```python
from build123d import *

# Parameters (mm, degrees)
SKETCH008_R       = 15
PAD004_DEPTH      = 3
PAD005_DEPTH      = 2
PAD005_DEPTH_BACK = 2
FILLET_R          = 2


with BuildPart() as part:
    # Sketch008 → Pad004 (new body)
    with BuildSketch(Plane.XY):
        Circle(SKETCH008_R)
    extrude(amount=PAD004_DEPTH)

    # Sketch009 → Pad005 (join, two sides)
    with BuildSketch(Plane.XZ) as pad005_sk:
        Polygon((-2, 0), (2, 0), (2, 24), (13.294118, 45.176471), (9.764706, 47.058824), (-2, 25), align=None)
    extrude(amount=PAD005_DEPTH)
    extrude(pad005_sk.sketch, amount=-PAD005_DEPTH_BACK)

    # Fillet
    fillet_edges = [part.edges().sort_by_distance(p)[0] for p in [
        (-15, 0, 3),
    ]]
    fillet(fillet_edges, radius=FILLET_R)


solid = part.part
```
For this review, take the finished solid that the model builds, in its own axes (mm). A direction names the side the tool comes from. Round coordinates to 2 decimals unless told otherwise and drop trailing zeros. Loops run counter-clockwise (first coordinate to the right, second up) from the corner with the lowest first, then second, coordinate; pieces in that order, holes last.
Q1. Insertion check: pin 1 Ø8 at (x, z) = (-2, 8.5) entering from +Y; pin 2 Ø4.5 at (x, z) = (3.5, 19) entering from -Y; pin 3 Ø1.2 at (y, z) = (-0.5, 17) entering from -X. Each pin has a flat end and moves straight along its axis. Give the tip position at first contact, or say it passes through.
Result sheet:
pin 1: stops at y = 2
pin 2: stops at y = -2
pin 3: stops at x = -2
Q2. Mouldability with a two-part tool opening along Z and no side actions: class faces 1 (the face through (3.965, 0.028, 36.184)), 2 (the face through (2, 2, 25)), 3 (the face through (2, 0, 13)) as +Z half, -Z half, draft (parallel to the pull), parting line (faces both ways), or undercut.
Result sheet:
face 1: +Z half
face 2: draft
face 3: undercut
Q3. Add section D-D on z = 30. Write out the cut boundary in (x, y).
Result sheet:
outline: (0.67, -2) - (5.2, -2) - (5.2, 2) - (0.67, 2) - close
Q4. Add section B-B on y = 0. Write out the cut boundary in (x, z).
Result sheet:
outline: (-15, 0) - (15, 0) - (15, 1) arc R2 ccw to (13, 3) - (2, 3) - (2, 24) - (13.29, 45.18) - (9.76, 47.06) - (-2, 25) - (-2, 3) - (-13, 3) arc R2 ccw to (-15, 1) - close
Q5. Add section C-C on z = 11.5. Write out the cut boundary in (x, y), plus the area to 3 significant figures.
Result sheet:
outline: (-2, -2) - (2, -2) - (2, 2) - (-2, 2) - close
area: 16.0 mm2
Q6. To check wall thickness, follow line 1 along Z through (x, y) = (-7.5, -5.5); line 2 along Y through (x, z) = (10, 43); line 3 along Z through (x, y) = (9, -0.25) (3 decimals). State the ranges of each line that lie inside material, in increasing order.
Result sheet:
line 1: z = 0 to 3
line 2: y = -2 to 2
line 3: z = 0 to 3, 37.125 to 45.625
Q7. Add section A-A on x = 0. Write out the cut boundary in (y, z).
Result sheet:
outline: (-15, 0) - (15, 0) - (15, 1) arc R2 ccw to (13, 3) - (2, 3) - (2, 28.75) - (-2, 28.75) - (-2, 3) - (-13, 3) arc R2 ccw to (-15, 1) - close
Q8. Machinability: for faces 4 (the face through (7.57, 0.03, 34.44)), 5 (the face through (11.554, 0.028, 46.104)), 6 (the face through (-2, 0, 14)), 7 (the face through (2, -2, 25)), which of the approach directions +Z, -Z, +X, -X, +Y, -Y give a long, thin tool a straight path to every point of the face, cutting with its end or side? Answer none if there is none.
Result sheet:
face 4: +X, +Y, -Y
face 5: +Z, +X, +Y, -Y
face 6: +Z, -X, +Y, -Y
face 7: +Z, +X, -X, -Y
